```python
from build123d import *

# Parameters (mm, degrees)
F0_R      = 2.2
F1_DEPTH  = 5
F5_W      = 7
F5_H      = 8
F6_DEPTH  = 8
F10_DEPTH = 7
F12_DEPTH = 22.94269
F13_W     = 1.95429
F13_H     = 8
F14_DEPTH = 1.5
F15_R     = 3
F16_R     = 3


with BuildPart() as f1:
    # F0 (on Front) → F1 (new body)
    with BuildSketch(Plane.XZ):
        with BuildLine():
            Line((-1.878526, 14.238436), (-25.570216, 4.633696))
            ThreePointArc((-25.570216, 4.633696), (-28.69169, 0), (-25.570216, -4.633696))
            Line((-25.570216, -4.633696), (-1.878526, -14.238436))
            ThreePointArc((-1.878526, -14.238436), (0, -14.604739), (1.878526, -14.238436))
            Line((1.878526, -14.238436), (25.570216, -4.633696))
            ThreePointArc((25.570216, -4.633696), (28.69169, 0), (25.570216, 4.633696))
            Line((25.570216, 4.633696), (1.878526, 14.238436))
            ThreePointArc((1.878526, 14.238436), (0, 14.604739), (-1.878526, 14.238436))
        make_face()
        with Locations((-23, 0)):
            Circle(F0_R, mode=Mode.SUBTRACT)
        Polygon((0, 6.639528), (5.75, 3.319764), (5.75, -3.319764), (0, -6.639528), (-5.75, -3.319764), (-5.75, 3.319764), align=None, mode=Mode.SUBTRACT)
        with Locations((23, 0)):
            Circle(F0_R, mode=Mode.SUBTRACT)
    extrude(amount=F1_DEPTH)

    # F3 (on Top) → F4 (revolve)
    with BuildSketch(Plane.XY):
        Polygon((-9, 0), (-12, 0), (-12, -7), (-8.809743, -13), (-7.25, -13), (-7.25, -10.291271), (-9, -7), align=None)
    revolve(axis=Axis((0, -6.211402, 0), (0, 1, 0)))

    # F5 (on face) → F6 (join)
    with BuildSketch(Plane.XZ.offset(5)):
        with Locations((-12.5, 0)):
            Rectangle(F5_W, F5_H)
    extrude(amount=F6_DEPTH)

    # F7 (on Top) → F8 (revolve, cut)
    with BuildSketch(Plane.XY):
        Polygon((-12, -13), (-9.7, -13), (-10.18, -5), (-12, -5), align=None)
    revolve(axis=Axis((-12, -9.796117, 0), (0, -1, 0)), mode=Mode.SUBTRACT)

    # F9 (on face) → F10 (cut)
    with BuildSketch(Plane.YZ.offset(-5.75)):
        Polygon((-8.434347, 0), (-5, -1.25), (-5, 1.25), align=None)
    extrude(amount=-F10_DEPTH, mode=Mode.SUBTRACT)

    # F11 (on face) → F12 (cut, through all)
    with BuildSketch(Plane(origin=(5.75, 0, 0), x_dir=(0, -1, 0), z_dir=(-1, 0, 0))):
        Polygon((7.060608, 0), (5, 0.75), (5, -0.75), align=None)
    extrude(amount=-F12_DEPTH, mode=Mode.SUBTRACT)

    # F13 (on face) → F14 (join)
    with BuildSketch(Plane.YZ.offset(-9)):
        with Locations((-12.022855, 0)):
            Rectangle(F13_W, F13_H)
    extrude(amount=F14_DEPTH)

    # F15
    f15_edges = [f1.edges().sort_by_distance(p)[0] for p in [
        (-16, -9, -4),
    ]]
    fillet(f15_edges, radius=F15_R)

    # F16
    f16_edges = [f1.edges().sort_by_distance(p)[0] for p in [
        (-16, -9, 4),
    ]]
    fillet(f16_edges, radius=F16_R)


solid = f1.part
```
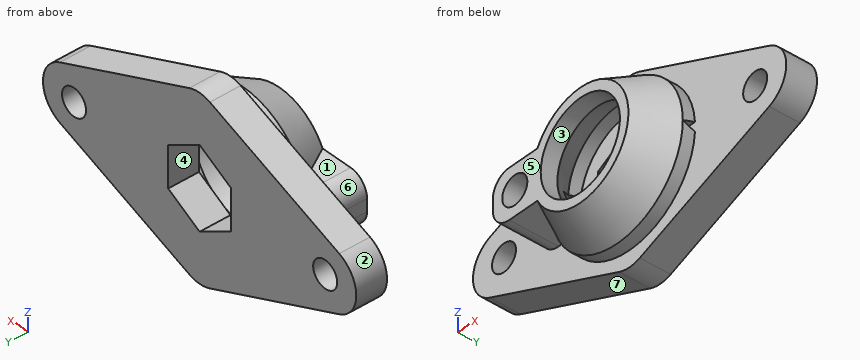
Source: CAD feature listing. Evaluate the final solid. Frame: model axes, mm. Face numbers are marked on the shaded views. A direction names the side the tool comes from. Coordinates: 2 decimals unless noted, no trailing zeros. Write each loop counter-clockwise with the first axis right and the second up, starting at its lowest first coordinate (ties: lowest second). Pieces come first, ordered by that corner, then holes. Notation, with made-up numbers: (-4, 37.25) - (14, 37.25) arc R18 cw to (14, 58.25) - close; hole circle Ø10 at (87, -1.5). An arc over 180 degrees is marked (long way). Answer as a JSON object with one key per item and string values.
Q1. First-contact query: pin 1 Ø2 at (x, z) = (-15, -8.5) entering from -Y; pin 2 Ø8.5 at (x, z) = (0, 0) entering from +Y; pin 3 Ø2 at (x, y) = (12, -3) entering from -Z; pin 4 Ø2 at (y, z) = (-9.5, 0) entering from -X. Flat tips, straight axial feed; report the tip coordinate or a pass-through.
Ans:
{"pin 1": "stops at y = -5", "pin 2": "passes through", "pin 3": "stops at z = -10.54", "pin 4": "stops at x = -16"}
Q2. Set-up query: the marked faces 1, 2 and 3. Return all of +Z, -Z, +X, -X, +Y, -Y with unobstructed straight access to the full face (end or side cutting, diameter ignored); none if empty.
Ans:
{"face 1": "+Z, -X, -Y", "face 2": "-X, +Y, -Y", "face 3": "-Y"}
Q3. Section query B-B, the plane x = 21.5. Output: boundary loops of the cut face in (y, z).
Ans:
{"outline": "(-5, -6.28) - (0, -6.28) - (0, -1.61) - (-5, -1.61) - close; (-5, 1.61) - (0, 1.61) - (0, 6.28) - (-5, 6.28) - close"}
Q4. Material intervals for line 1 (X direction, y = -8.5, z = -6.5); line 2 (Z direction, x = 23, y = -3.8); line 3 (X direction, y = -6.75, z = 5.5), sorted ascending. Write a range as [from, to].
Ans:
{"line 1": "x = [-9.12, -5], [5, 9.12]", "line 2": "z = [-5.68, -2.2], [2.2, 5.68]", "line 3": "x = [-10.67, -7.12], [7.12, 10.67]"}
Q5. Section query A-A, the plane y = -1. Output: boundary loops of the cut face in (x, z).
Ans:
{"outline": "(-25.57, -4.63) - (-1.88, -14.24) arc R5 ccw to (1.88, -14.24) - (25.57, -4.63) arc R5 ccw to (25.57, 4.63) - (1.88, 14.24) arc R5 ccw to (-1.88, 14.24) - (-25.57, 4.63) arc R5 ccw to start; hole circle Ø4.4 at (-23, 0); hole (-5.75, -3.32) - (0, -6.64) - (5.75, -3.32) - (5.75, 3.32) - (0, 6.64) - (-5.75, 3.32) - close; hole circle Ø4.4 at (23, 0)"}
Q6. Draft query along Z for the marked faces 4, 5, 6 and 7. Return one class per face: released by +Z, released by -Z, zero draft, split by the parting line, or undercut.
Ans:
{"face 4": "undercut", "face 5": "zero draft", "face 6": "released by +Z", "face 7": "released by -Z"}
Q7. Section query C-C, the plane x = -12. Output: boundary loops of the cut face in (y, z).
Ans:
{"outline": "(-13, -4) - (-5, -4) - (-5, -10.14) - (0, -10.14) - (0, 10.14) - (-5, 10.14) - (-5, 4) - (-13, 4) - (-13, 2.3) - (-5, 1.82) - (-5, -1.82) - (-13, -2.3) - close"}
Q8. Section query D-D, the plane x = -24. Output: boundary loops of the cut face in (y, z), plus the area to 3 significant figures.
Ans:
{"outline": "(-5, -5.27) - (0, -5.27) - (0, -1.96) - (-5, -1.96) - close; (-5, 1.96) - (0, 1.96) - (0, 5.27) - (-5, 5.27) - close", "area": "33.1 mm2"}
